For this review, use the dimensioned drawing (mm, ordinates from the lowest corner) and the shaded views. Round coordinates to 2 decimals unless told otherwise and drop trailing zeros. Loops run counter-clockwise (first coordinate to the right, second up) from the corner with the lowest first, then second, coordinate; pieces in that order, holes last. Notation, with made-up numbers: (71, 18.25) -> (125, 18.25) arc R17 ccw to (125, 49.25) -> close; hole circle Ø4 at (88.25, -35). An arc over 180 degrees is marked (long way). Use one line per item in the form item = value. Start each with the question number.
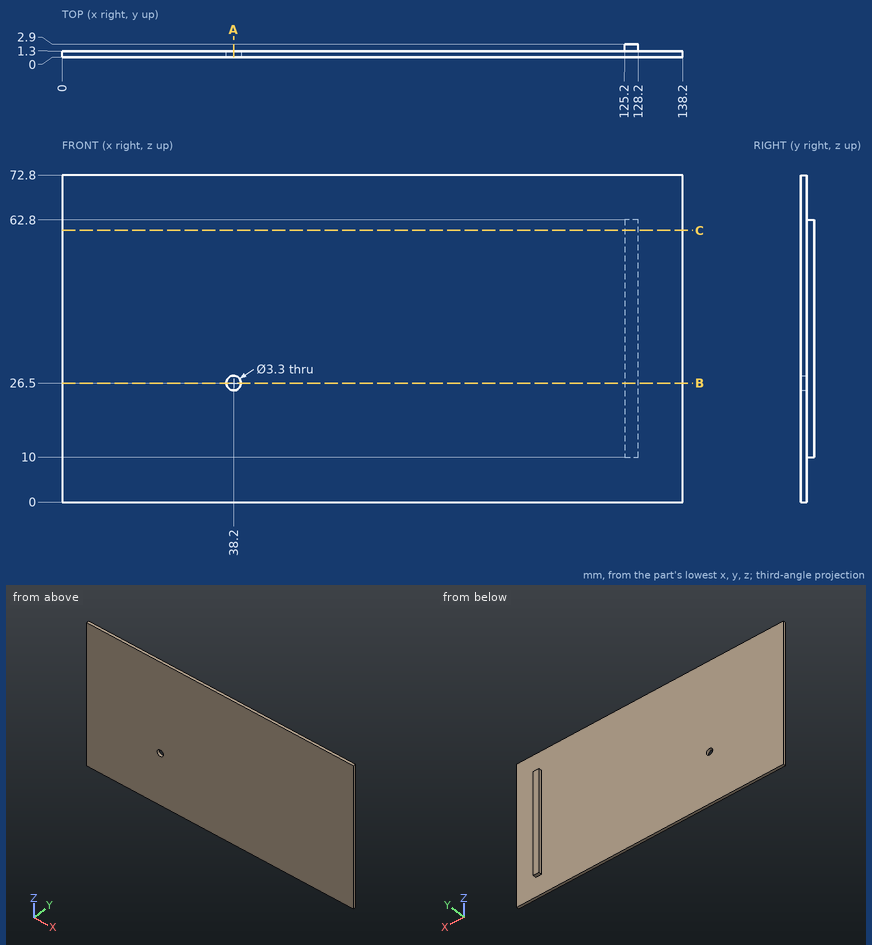
Item 1: Take a section at B-B on z = 26.5. Give the boundary of the cut face in (x, y).
Item 2: Wall thickness on line 1 (X direction, y = 0.8, z = 26.5); line 2 (Z direction, x = 38.2, y = 0.6); line 3 (X direction, y = 1.8, z = 62.5): over which ranges is each line inside the solid? List them lowest first.
Item 3: Take a section at C-C on z = 60.5. Give the boundary of the cut face in (x, y), plus the area to 3 significant figures.
Item 4: For P1, Ø0.5, axis at y = 2, z = 44, coming from the -X side; P2, Ø0.5, axis at y = 2, z = 32, coming from the +X side; P3, Ø1.5, axis at x = 60.5, z = 49.5, coming from the +Y side; P4, Ø2, axis at x = 38.2, z = 26.5, coming from the -Y side, all flat-tipped, find the tip position at first contact; note any pin that passes through.
Item 5: Take a section at A-A on x = 38.2. Give the boundary of the cut face in (y, z).
Results:
q1.outline = (0, 0) -> (36.55, 0) -> (36.55, 1.3) -> (0, 1.3) -> close; (39.85, 0) -> (138.2, 0) -> (138.2, 1.3) -> (128.2, 1.3) -> (128.2, 2.9) -> (125.2, 2.9) -> (125.2, 1.3) -> (39.85, 1.3) -> close
q2.line_1 = 0 to 36.55, 39.85 to 138.2
q2.line_2 = 0 to 24.85, 28.15 to 72.8
q2.line_3 = 125.2 to 128.2
q3.outline = (0, 0) -> (138.2, 0) -> (138.2, 1.3) -> (128.2, 1.3) -> (128.2, 2.9) -> (125.2, 2.9) -> (125.2, 1.3) -> (0, 1.3) -> close
q3.area = 184 mm2
q4.P1 = 125.2
q4.P2 = 128.2
q4.P3 = 1.3
q4.P4 = through
q5.outline = (0, 0) -> (1.3, 0) -> (1.3, 24.85) -> (0, 24.85) -> close; (0, 28.15) -> (1.3, 28.15) -> (1.3, 72.8) -> (0, 72.8) -> close
